```python
from build123d import *

# Parameters (mm, degrees)
PAD005_DEPTH            = 8.1
POCKET003_DEPTH         = 7
SKETCH010_W             = 6.8
SKETCH010_H             = 5
POCKET004_DEPTH         = 1
SKETCH011_W             = 5.5
SKETCH011_H             = 3
POCKET005_DEPTH         = 3
PAD006_DEPTH            = 4
PAD014_DEPTH            = 3.4
BODY005_PLACEMENT_ANGLE = 180


with BuildPart() as part:
    # Sketch008 → Pad005 (new body)
    with BuildSketch(Plane.XY):
        Polygon((-5, 0), (-3.05, 0), (-3.05, 1), (3.05, 1), (3.05, 0), (5, 0), (5, 5.1), (-5, 5.1), align=None)
    extrude(amount=PAD005_DEPTH)

    # Sketch009 (on Face10 of Pad005) → Pocket003 (cut)
    with BuildSketch(Plane.XY.offset(8.1)):
        Polygon((-4.45, 0.55), (-3.45, 0.55), (-3.45, 1.55), (3.45, 1.55), (3.45, 0.55), (4.45, 0.55), (4.45, 4.55), (-4.45, 4.55), align=None)
    extrude(amount=-POCKET003_DEPTH, mode=Mode.SUBTRACT)

    # Sketch010 (on Face5 of Pocket003) → Pocket004 (cut)
    with BuildSketch(Plane.XY.offset(8.1)):
        with Locations((0, 5.5)):
            Rectangle(SKETCH010_W, SKETCH010_H)
    extrude(amount=-POCKET004_DEPTH, mode=Mode.SUBTRACT)

    # Sketch011 (on Face5 of Pocket004) → Pocket005 (cut)
    with BuildSketch(Plane.XY.offset(8.1)):
        with Locations((0, 1.5)):
            Rectangle(SKETCH011_W, SKETCH011_H)
    extrude(amount=-POCKET005_DEPTH, mode=Mode.SUBTRACT)

    # Sketch012 (on Face26 of Pocket005) → Pad006 (join)
    with BuildSketch(Plane.XY.offset(1.1)):
        with BuildLine():
            ThreePointArc((-3.4, 3.25), (-3.65, 3), (-3.4, 2.75))
            Line((-3.4, 2.75), (3.4, 2.75))
            ThreePointArc((3.4, 2.75), (3.65, 3), (3.4, 3.25))
            Line((-3.4, 3.25), (3.4, 3.25))
        make_face()
    extrude(amount=PAD006_DEPTH)

    # Sketch020 (on Face4 of Pad006) → Pad014 (join)
    with BuildSketch(Plane(origin=(0, 0, 0), x_dir=(1, 0, 0), z_dir=(0, 0, -1))):
        with BuildLine():
            ThreePointArc((-3, -2.25), (-3.75, -3), (-3, -3.75))
            Line((-3, -3.75), (3, -3.75))
            ThreePointArc((3, -3.75), (3.75, -3), (3, -2.25))
            Line((-3, -2.25), (3, -2.25))
        make_face()
    extrude(amount=PAD014_DEPTH)


with BuildPart() as part_1:
    # Body005 placement: moved
    add(part.part.moved(Location((-7, 29, 0))).rotate(Axis((-7, 29, 0), (0, 0, 1)), BODY005_PLACEMENT_ANGLE))


with BuildPart() as part_2:
    # Body012 placement: moved
    add(part_1.part.moved(Location((14, 26, 0))))


solid = part_2.part
```
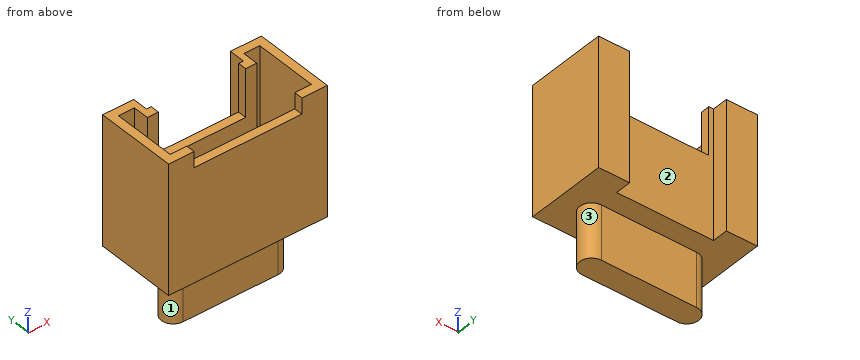
For this review, take the finished solid that the model builds, in its own axes (mm). Face numbers are marked on the shaded views. A direction names the side the tool comes from. Coordinates: 2 decimals unless noted, no trailing zeros. Write each loop counter-clockwise with the first axis right and the second up, starting at its lowest first coordinate (ties: lowest second). Pieces come first, ordered by that corner, then holes.
(1) Add section A-A on y = 52.6. Give the boundary of the cut face in (x, z), then the cut area to 3 significant figures.
(2) Add section D-D on y = 50.75. Give the boundary of the cut face in (x, z), then the cut area to 3 significant figures.
(3) Tool access review of the marked faces 1, 2 and 3: name each direction out of +Z, -Z, +X, -X, +Y, -Y from which nothing blocks a thin tool from reaching the whole face with its end or side.
(4) Add section B-B on z = 0.5. Give the boundary of the cut face in (x, y).
(5) Wall thickness on probe 1 along X at (y, z) = (54.4, 5); probe 2 along Y at (x, z) = (9, 2.5); probe 3 along X at (y, z) = (53.65, 5.5): over which ranges is each line inside the solid? List them lowest first.
(6) For pin 1 Ø1 at (y, z) = (53, -1) entering from +X; pin 2 Ø1.8 at (x, z) = (7, 3.5) entering from +Y; pin 3 Ø1.5 at (x, y) = (7, 54) entering from +Z; pin 4 Ø3.5 at (x, z) = (7, -1) entering from -Y, all flat-tipped, find the tip position at first contact; note any pin that passes through.
(7) Add section C-C on x = 9.5. Give the boundary of the cut face in (y, z).
Answer sheet:
1. outline: (2, 0) - (3.55, 0) - (3.55, -3.4) - (10.45, -3.4) - (10.45, 0) - (12, 0) - (12, 8.1) - (11.45, 8.1) - (11.45, 1.1) - (2.55, 1.1) - (2.55, 8.1) - (2, 8.1) - close
1. area: 42.2 mm2
2. outline: (2, 0) - (12, 0) - (12, 8.1) - (11.45, 8.1) - (11.45, 1.1) - (2.55, 1.1) - (2.55, 8.1) - (2, 8.1) - close
2. area: 18.7 mm2
3. face 1: -Z, -X
3. face 2: +Z, -Z, +Y
3. face 3: -Z, +X
4. outline: (2, 49.9) - (12, 49.9) - (12, 55) - (10.05, 55) - (10.05, 54) - (3.95, 54) - (3.95, 55) - (2, 55) - close
5. probe 1: x = 2 to 2.55, 3.55 to 3.95, 10.05 to 10.45, 11.45 to 12
5. probe 2: y = 49.9 to 50.45, 51.75 to 52.25, 53.45 to 54
5. probe 3: x = 2 to 2.55, 3.55 to 4.25, 9.75 to 10.45, 11.45 to 12
6. pin 1: stops at x = 10.56
6. pin 2: stops at y = 54
6. pin 3: stops at z = 5.1
6. pin 4: stops at y = 49.9
7. outline: (49.9, 0) - (51.25, 0) - (51.25, -3.4) - (52.75, -3.4) - (52.75, 0) - (54, 0) - (54, 5.1) - (53.45, 5.1) - (53.45, 1.1) - (52.25, 1.1) - (52.25, 5.1) - (51.75, 5.1) - (51.75, 1.1) - (50.45, 1.1) - (50.45, 7.1) - (49.9, 7.1) - close
